Could you check a few things on this model? Use its own coordinates, in mm. Face numbers are marked on the shaded views. A direction names the side the tool comes from. Coordinates: 2 decimals unless noted, no trailing zeros. Write each loop counter-clockwise with the first axis right and the second up, starting at its lowest first coordinate (ties: lowest second). Pieces come first, ordered by that corner, then holes.
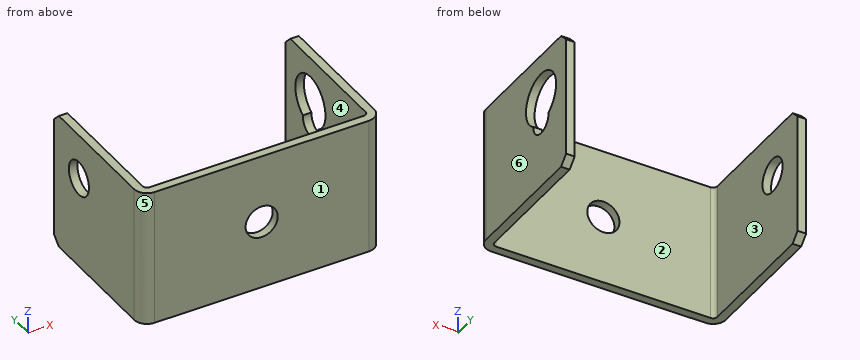
```python
from build123d import *

# Parameters (mm, degrees)
BASE_FLANGE1_DEPTH = 32
CUT_EXTRUDE1_DEPTH = 10
SKETCH7_R          = 4
CUT_EXTRUDE2_DEPTH = 10
SKETCH8_R          = 3.75
CUT_EXTRUDE4_DEPTH = 10
CHAMFER1_SIZE      = 2


# Read off the part's stored shape, not the designer's step: Base-Flange1
with BuildPart() as part:
    # Base-Flange1 outline → Base-Flange1 (new body)
    with BuildSketch(Plane.XY):
        with BuildLine():
            Line((56, 3), (56, 35))
            Line((56, 35), (54, 35))
            Line((54, 35), (54, 3))
            ThreePointArc((54, 3), (53.707106781, 2.292893219), (53, 2))
            Line((53, 2), (3, 2))
            ThreePointArc((3, 2), (2.292893219, 2.292893219), (2, 3))
            Line((2, 3), (2, 35))
            Line((2, 35), (0, 35))
            Line((0, 35), (0, 3))
            ThreePointArc((0, 3), (0.878679656, 0.878679656), (3, 0))
            Line((3, 0), (53, 0))
            ThreePointArc((53, 0), (55.121320344, 0.878679656), (56, 3))
        make_face()
    extrude(amount=BASE_FLANGE1_DEPTH)

    # Sketch6 → Cut-Extrude1 (cut)
    with BuildSketch(Plane(origin=(56, 0, 0), x_dir=(0, 0, -1), z_dir=(1, 0, 0))):
        with BuildLine():
            ThreePointArc((-16.295454545, 27.985415651), (-27.5, 25), (-16.295454545, 22.014584349))
            ThreePointArc((-16.295454545, 22.014584349), (-13, 25), (-16.295454545, 27.985415651))
        make_face()
    extrude(amount=-CUT_EXTRUDE1_DEPTH, mode=Mode.SUBTRACT)

    # Sketch7 → Cut-Extrude2 (cut)
    with BuildSketch(Plane.ZY):
        with Locations((21.5, 25)):
            Circle(SKETCH7_R)
    extrude(amount=-CUT_EXTRUDE2_DEPTH, mode=Mode.SUBTRACT)

    # Sketch8 → Cut-Extrude4 (cut)
    with BuildSketch(Plane(origin=(0, 2, 0), x_dir=(1, 0, 0), z_dir=(0, 1, 0))):
        with Locations(Location((28, -16, 0), (0, 0, 270))):
            Circle(SKETCH8_R)
    extrude(amount=-CUT_EXTRUDE4_DEPTH, mode=Mode.SUBTRACT)

    # Chamfer1
    chamfer1_edges = [part.edges().sort_by_distance(p)[0] for p in [
        (1, 35, 0),
        (55, 35, 0),
        (1, 35, 32),
        (55, 35, 32),
    ]]
    chamfer(chamfer1_edges, length=CHAMFER1_SIZE)


solid = part.part
```
1. I want a section at D-D on z = 15. Please give me the cut outline in (x, y).
Verdict:
outline: (0, 3) arc R3 ccw to (3, 0) - (24.39, 0) - (24.39, 2) - (3, 2) arc R1 cw to (2, 3) - (2, 35) - (0, 35) - close; (31.61, 0) - (53, 0) arc R3 ccw to (56, 3) - (56, 22.17) - (54, 22.17) - (54, 3) arc R1 cw to (53, 2) - (31.61, 2) - close; (54, 27.83) - (56, 27.83) - (56, 35) - (54, 35) - close
2. On a 3-axis mill with a long thin cutter (end or side, diameter ignored), from which of +Z, -Z, +X, -X, +Y, -Y can I reach the whole of each face in a straight line? I mean the marked faces 1 and 2. Say none if no direction works.
Verdict:
face 1: +Z, -Z, +X, -X, -Y
face 2: +Z, -Z, +Y
3. For pin 1 (3.5 mm diameter, centred on y = 25, z = 16, fed in from +X); pin 2 (9.5 mm diameter, centred on x = 36, z = 20.5, fed in from +Y); pin 3 (5 mm diameter, centred on y = 25, z = 21.5, fed in from +X), each with a flat end and sliding along its axis, tell me the tip position at first contact or that it passes through.
Verdict:
pin 1: stops at x = 2
pin 2: stops at y = 2
pin 3: passes through
4. I want a section at A-A on z = 21.5. Please give me the cut outline in (x, y).
Verdict:
outline: (0, 3) arc R3 ccw to (3, 0) - (53, 0) arc R3 ccw to (56, 3) - (56, 19) - (54, 19) - (54, 3) arc R1 cw to (53, 2) - (3, 2) arc R1 cw to (2, 3) - (2, 21) - (0, 21) - close; (0, 29) - (2, 29) - (2, 35) - (0, 35) - close; (54, 31) - (56, 31) - (56, 35) - (54, 35) - close
5. I want a section at C-C on y = 7.5. Please give me the cut outline in (x, z), plus the area to 3 significant figures.
Verdict:
outline: (0, 0) - (2, 0) - (2, 32) - (0, 32) - close; (54, 0) - (56, 0) - (56, 32) - (54, 32) - close
area: 128 mm2
6. I want a section at B-B on y = 25. Please give me the cut outline in (x, z).
Verdict:
outline: (0, 0) - (2, 0) - (2, 17.5) - (0, 17.5) - close; (0, 25.5) - (2, 25.5) - (2, 32) - (0, 32) - close; (54, 0) - (56, 0) - (56, 13) - (54, 13) - close; (54, 27.5) - (56, 27.5) - (56, 32) - (54, 32) - close
7. If we mould it in two halves opening along X, with no side actions, what happens to the marked faces 3, 4, 5 and 6? For each: pulls with the +X half, pulls with the -X half, needs draft (parallel to the pull), parting line crosses it, or undercut.
Verdict:
face 3: undercut
face 4: undercut
face 5: pulls with the -X half
face 6: pulls with the +X half
8. Please list where these lines run through material, in increasing order: line 1 along X through (y, z) = (5, 10.5); line 2 along Y through (x, z) = (23.5, 18.5); line 3 along Y through (x, z) = (54.4, 16).
Verdict:
line 1: x = 0 to 2, 54 to 56
line 2: y = 0 to 2
line 3: y = 0.35 to 22, 28 to 35
